```python
from build123d import *

# Parameters (mm, degrees)
SKETCH1_R           = 5.8
BOSS_EXTRUDE1_DEPTH = 5
SKETCH2_R           = 3.5
CUT_EXTRUDE1_DEPTH  = 3.5
SKETCH3_R           = 8.275638688
SKETCH3_R_2         = 5.05
CUT_EXTRUDE2_DEPTH  = 3


with BuildPart() as part:
    # Sketch1 → Boss-Extrude1 (new body)
    with BuildSketch(Plane(origin=(0, 0, 0), x_dir=(1, 0, 0), z_dir=(0, 1, 0))):
        with Locations(Location((0, 0, 0), (0, 0, 270))):
            Circle(SKETCH1_R)
    extrude(amount=BOSS_EXTRUDE1_DEPTH)

    # Sketch2 → Cut-Extrude1 (cut)
    with BuildSketch(Plane(origin=(0, 5, 0), x_dir=(1, 0, 0), z_dir=(0, 1, 0))):
        with Locations(Location((0, 0, 0), (0, 0, 270))):
            Circle(SKETCH2_R)
    extrude(amount=-CUT_EXTRUDE1_DEPTH, mode=Mode.SUBTRACT)

    # Sketch3 → Cut-Extrude2 (cut)
    with BuildSketch(Plane(origin=(0, 5, 0), x_dir=(1, 0, 0), z_dir=(0, 1, 0))):
        Circle(SKETCH3_R)
        with Locations(Location((0, 0, 0), (0, 0, 270))):
            Circle(SKETCH3_R_2, mode=Mode.SUBTRACT)
    extrude(amount=-CUT_EXTRUDE2_DEPTH, mode=Mode.SUBTRACT)


solid = part.part
```
CAD build for the part. Positions are in the model's coordinates, mm. A direction names the side the tool comes from. Coordinates: 2 decimals unless noted, no trailing zeros. Write each loop counter-clockwise with the first axis right and the second up, starting at its lowest first coordinate (ties: lowest second). Pieces come first, ordered by that corner, then holes.
(1) Flat gauge pins, fed straight in: pin 1 (2 mm diameter, centred on x = -4.5, z = 1.5, fed in from -Y); pin 2 (1.5 mm diameter, centred on x = -1, z = -1, fed in from +Y); pin 3 (2 mm diameter, centred on x = -1.5, y = 2, fed in from -Z); pin 4 (1 mm diameter, centred on x = 4.5, y = 4, fed in from -Z). Where does each tip first touch, or does it go through?
(2) Two-plate mould, pull along X, no slides. Class faces 3 (the face through (-3.417, 3.274, -0.759)), 4 (the face through (-2, 2, -5)), 5 (the face through (-3.07, 3.52, -4.01)): +X half, -X half, draft (parallel to the pull), parting line (faces both ways), or undercut.
(3) Drill centre lines: probe 1 along X at (y, z) = (3.2, 0); probe 2 along Y at (x, z) = (-0.75, -0.75); probe 3 along X at (y, z) = (3.15, -0.75). Where is each one in solid material? Low to high.
(4) Cut at B-B, the plane x = 0. List the corners of the cut face in (y, z).
(5) Cut at A-A, the plane z = 0. List the corners of the cut face in (x, y), and give its area (3 significant figures).
(6) Cut at D-D, the plane y = 0.5. List the corners of the cut face in (x, z), and give its area (3 significant figures).
(7) 3-axis set-ups, long thin cutter, end or side, ignore diameter. For faces 1 (the face through (0.255, 0.986, -5.794)), 2 (the face through (0, 1.5, 0)): which of +Z, -Z, +X, -X, +Y, -Y reach the whole face in a straight line?
(8) Cut at C-C, the plane y = 2.5. List the corners of the cut face in (x, z).
Geometry says:
1. pin 1: stops at y = 0
1. pin 2: stops at y = 1.5
1. pin 3: stops at z = -5.78
1. pin 4: stops at z = -3.08
2. face 3: undercut
2. face 4: draft
2. face 5: parting line
3. probe 1: x = -5.05 to -3.5, 3.5 to 5.05
3. probe 2: y = 0 to 1.5
3. probe 3: x = -4.99 to -3.42, 3.42 to 4.99
4. outline: (0, -5.8) - (2, -5.8) - (2, -5.05) - (5, -5.05) - (5, -3.5) - (1.5, -3.5) - (1.5, 3.5) - (5, 3.5) - (5, 5.05) - (2, 5.05) - (2, 5.8) - (0, 5.8) - close
5. outline: (-5.8, 0) - (5.8, 0) - (5.8, 2) - (5.05, 2) - (5.05, 5) - (3.5, 5) - (3.5, 1.5) - (-3.5, 1.5) - (-3.5, 5) - (-5.05, 5) - (-5.05, 2) - (-5.8, 2) - close
5. area: 29.0 mm2
6. outline: circle Ø11.6 at (0, 0)
6. area: 106 mm2
7. face 1: +Y, -Y
7. face 2: +Y
8. outline: circle Ø10.1 at (0, 0); hole circle Ø7 at (0, 0)
